Autodesk Inventor part; units mm, degrees
ref_plane "YZ Plane" through (0, 0, 0) normal (1, 0, 0) x (0, 1, 0)
ref_plane "XZ Plane" through (0, 0, 0) normal (0, 1, 0) x (-1, 0, 0)
ref_plane "XY Plane" through (0, 0, 0) normal (0, 0, 1) x (1, 0, 0)
sketch "Sketch1" plane through (0, 0, 0) normal (0, 0, 1) x (1, 0, 0)
  circle A0 centre (10, -42.5) radius 5.5
  circle A1 centre (10, 42.5) radius 5.5
  circle A2 centre (32, -42.5) radius 5.5
  circle A3 centre (32, 42.5) radius 5.5
  line L0 (42, -50.5) -> (42, 50.5)
  line L1 (0, 50.5) -> (42, 50.5)
  line L2 (0, 50.5) -> (0, -50.5)
  line L3 (0, -50.5) -> (42, -50.5)
  point P0 (0, 0)
extrude "Extrusion1" add sketch "Sketch1" along normal blind 43
properties part number "BaseBallScrewSupport"
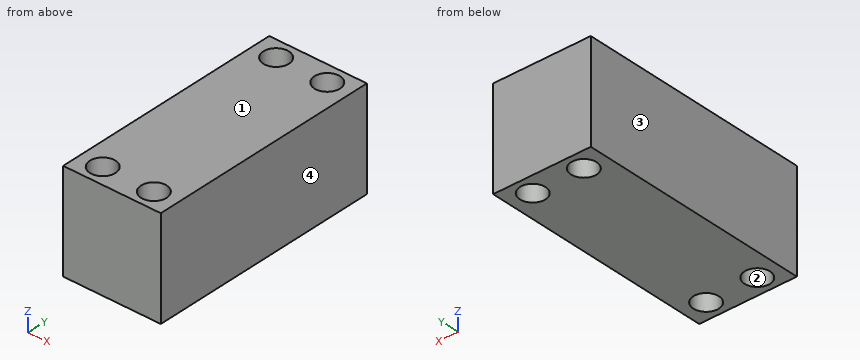
Verification items for the finished model (mm, model axes). Face numbers are marked on the shaded views. Coordinates: 2 decimals unless noted, no trailing zeros. Write each loop counter-clockwise with the first axis right and the second up, starting at its lowest first coordinate (ties: lowest second). Pieces come first, ordered by that corner, then holes. Notation, with made-up numbers: (47, 57) - (73, 57) arc R37 cw to (73, 95) - close; hole circle Ø9 at (72.25, 41.25). An arc over 180 degrees is marked (long way). Answer as a JSON object with one key per item and string values.
(1) Cross-section at B-B on z = 25. Record the cut outline in (x, y).
Report:
{"outline": "(0, -50.5) - (42, -50.5) - (42, 50.5) - (0, 50.5) - close; hole circle Ø11 at (10, -42.5); hole circle Ø11 at (10, 42.5); hole circle Ø11 at (32, -42.5); hole circle Ø11 at (32, 42.5)"}
(2) Thickness scan on line 1 along Y through (x, z) = (10, 32); line 2 along Y through (x, z) = (35, 20); line 3 along X through (y, z) = (42, 14). Record the ranges inside material, lowest first.
Report:
{"line 1": "-50.5 to -48, -37 to 37, 48 to 50.5", "line 2": "-50.5 to -47.11, -37.89 to 37.89, 47.11 to 50.5", "line 3": "0 to 4.52, 15.48 to 26.52, 37.48 to 42"}
(3) Mould release check, pull along X, two halves, no side actions. Record for the marked faces 1, 2, 3 and 4: pulls with the +X half, pulls with the -X half, needs draft (parallel to the pull), parting line crosses it, or undercut.
Report:
{"face 1": "needs draft", "face 2": "undercut", "face 3": "pulls with the -X half", "face 4": "pulls with the +X half"}
(4) Cross-section at A-A on y = 42.5. Record the cut outline in (x, z).
Report:
{"outline": "(0, 0) - (4.5, 0) - (4.5, 43) - (0, 43) - close; (15.5, 0) - (26.5, 0) - (26.5, 43) - (15.5, 43) - close; (37.5, 0) - (42, 0) - (42, 43) - (37.5, 43) - close"}
(5) Cross-section at C-C on x = 10. Record the cut outline in (y, z), plus the area to 3 significant figures.
Report:
{"outline": "(-50.5, 0) - (-48, 0) - (-48, 43) - (-50.5, 43) - close; (-37, 0) - (37, 0) - (37, 43) - (-37, 43) - close; (48, 0) - (50.5, 0) - (50.5, 43) - (48, 43) - close", "area": "3,400 mm^2"}
